Could you check a few things on this model? Use its own coordinates, in mm. Face numbers are marked on the shaded views. A direction names the side the tool comes from. Round coordinates to 2 decimals unless told otherwise and drop trailing zeros. Write each loop counter-clockwise with the first axis right and the second up, starting at its lowest first coordinate (ties: lowest second). Pieces come first, ordered by that corner, then holes. Notation, with made-up numbers: (60.5, 69.5) -> (103.5, 69.5) arc R26 cw to (103.5, 83.5) -> close; hole circle Ø4 at (68.5, -34). An arc over 180 degrees is marked (long way). Answer in a Markdown table with one row per item. Add a question column.
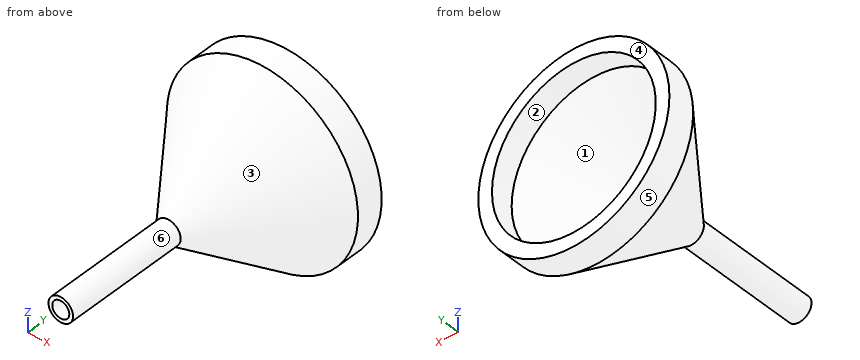
```python
from build123d import *

# Parameters (mm, degrees)
CROQUIS2_R            = 6.249824167
CORTAR_EXTRUIR1_DEPTH = 150


# Read off the part's stored shape, not the designer's step: Vaciado4
with BuildPart() as part:
    # Croquis1 → Revolución2 (revolve)
    with BuildSketch(Plane.XY, mode=Mode.PRIVATE) as revoluci_n2_sk:
        Polygon((0, 95), (0, -95), (9, -95), (9, -4.240141343), (70, 75), (70, 95), align=None)
    revolve(revoluci_n2_sk.sketch.rotate(Axis((0, 95, 0), (0, -1, 0)), 180), axis=Axis((0, 95, 0), (0, -1, 0)))

    # Vaciado4 outline → Vaciado4 (revolve, cut)
    with BuildSketch(Plane.XY):
        Polygon((0, 95), (0, 0.462132886), (60, 78.403255518), (60, 95), align=None)
    revolve(axis=Axis((0, 0, 0), (0, 1, 0)), mode=Mode.SUBTRACT)

    # Croquis2 → Cortar-Extruir1 (cut)
    with BuildSketch(Plane.XZ.offset(95)):
        Circle(CROQUIS2_R)
    extrude(amount=-CORTAR_EXTRUIR1_DEPTH, mode=Mode.SUBTRACT)


solid = part.part
```
(1) Suppose I cut it at A-A, the plane x = 0. Please give me the cut outline in (y, z).
(2) Suppose I cut it at D-D, the plane y = 33.5. Please give me the cut outline in (x, z).
(3) On a 3-axis mill with a long thin cutter (end or side, diameter ignored), from which of +Z, -Z, +X, -X, +Y, -Y can I reach the whole of each face in a straight line? I mean the marked faces 5 and 6. Say none if no direction works.
(4) Suppose I cut it at C-C, the plane y = -68. Please give me the cut outline in (x, z).
(5) Suppose I cut it at B-B, the plane z = 0. Please give me the cut outline in (x, y).
(6) If we mould it in two halves opening along X, with no side actions, what happens to the marked faces 1, 2, 3 and 4? For each: pulls with the +X half, pulls with the -X half, needs draft (parallel to the pull), parting line crosses it, or undercut.
(7) I need wall thicknesses on L1, parallel to Z at x = 0, y = 88.5; L2, parallel to Z at x = 0, y = -21; L3, parallel to X at y = 43, z = 16. Which ranges of each line are inside material? Lowest first, please.
(8) For P1, Ø6, axis at x = 0, y = -75, coming from the +Z side; P2, Ø1.5, axis at x = 19.5, z = 0.5, coming from the -Y side; P3, Ø4, axis at y = 15.5, z = 2.5, coming from the +X side, each with a flat end and sliding along its axis, tell me the tip position at first contact or that it passes through.
Response:
| question | item | result |
|---|---|---|
| 1 | outline | (-95, -9) -> (-4.24, -9) -> (75, -70) -> (95, -70) -> (95, -60) -> (78.4, -60) -> (8.58, -6.25) -> (-95, -6.25) -> close; (-95, 6.25) -> (8.58, 6.25) -> (78.4, 60) -> (95, 60) -> (95, 70) -> (75, 70) -> (-4.24, 9) -> (-95, 9) -> close |
| 2 | outline | circle Ø76.11 at (0, 0); hole circle Ø50.87 at (0, 0) |
| 3 | face 5 | +Y, -Y |
| 3 | face 6 | -Y |
| 4 | outline | circle Ø18 at (0, 0); hole circle Ø12.5 at (0, 0) |
| 5 | outline | (-70, 75) -> (-9, -4.24) -> (-9, -95) -> (-6.25, -95) -> (-6.25, 8.58) -> (-60, 78.4) -> (-60, 95) -> (-70, 95) -> close; (6.25, -95) -> (9, -95) -> (9, -4.24) -> (70, 75) -> (70, 95) -> (60, 95) -> (60, 78.4) -> (6.25, 8.58) -> close |
| 6 | face 1 | undercut |
| 6 | face 2 | undercut |
| 6 | face 3 | parting line crosses it |
| 6 | face 4 | needs draft |
| 7 | L1 | -70 to -60, 60 to 70 |
| 7 | L2 | -9 to -6.25, 6.25 to 9 |
| 7 | L3 | -42.45 to -28.57, 28.57 to 42.45 |
| 8 | P1 | z = 9 |
| 8 | P2 | y = 8.43 |
| 8 | P3 | x = 25.63 |
